```python
from build123d import *

# Parameters (mm, degrees)
SKETCH_1_W                = 300
SKETCH_1_H                = 300
EXTRUDE_1_DEPTH           = 4
EXTRUDE_2_DEPTH           = 76
FILLET_1_R                = 3
CUT_EXTRUDE_1_DEPTH       = 345.818792991
CUT_EXTRUDE_1_DEPTH_BACK  = 345.818792991
SKETCH_3_R                = 3
SKETCH_3_R_2              = 19.5
SKETCH_4_W                = 6
SKETCH_4_H                = 300
EXTRUDE_3_DEPTH           = 76
SKETCH_7_R                = 2
CUT_EXTRUDE_3_DEPTH       = 10
SKETCH_14_W               = 80
SKETCH_14_H               = 30
CUT_EXTRUDE_9_DEPTH       = 20
CUT_EXTRUDE_10_DEPTH      = 345.818792991
CUT_EXTRUDE_10_DEPTH_BACK = 345.818792991
SKETCH_15_R               = 3.5
SKETCH_16_W               = 4
SKETCH_16_H               = 288
EXTRUDE_5_DEPTH           = 9
CHAMFER_3_SIZE            = 50
SKETCH_17_R               = 2.25
SKETCH_17_R_2             = 2.5
CUT_EXTRUDE_11_DEPTH      = 6
SKETCH_18_W               = 137.872576177
SKETCH_18_H               = 47.95567867
SKETCH_18_W_2             = 92.314681441
SKETCH_18_H_2             = 203.212188366
SKETCH_18_W_3             = 138.671837489
SKETCH_18_H_3             = 133.676454294
SKETCH_18_H_4             = 48.754939981
CUT_EXTRUDE_12_DEPTH      = 6
FILLET_4_R                = 3


with BuildPart() as part:
    # Эскиз1 → Бобышка-Вытянуть1 (new body)
    with BuildSketch(Plane(origin=(0, 0, 0), x_dir=(1, 0, 0), z_dir=(0, 1, 0))):
        Rectangle(SKETCH_1_W, SKETCH_1_H)
    extrude(amount=EXTRUDE_1_DEPTH)

    # Эскиз2 → Бобышка-Вытянуть2 (add)
    with BuildSketch(Plane(origin=(0, 4, 0), x_dir=(1, 0, 0), z_dir=(0, 1, 0))):
        Polygon((150, 150), (-144, 150), (-144, 144), (144, 144), (144, -144), (-144, -144), (-144, -150), (150, -150), (150, 0.239524614), align=None)
    extrude(amount=EXTRUDE_2_DEPTH)

    # Скругление1
    fillet_1_edges = [part.edges().sort_by_distance(p)[0] for p in [
        (150, 40, 150),
        (150, 40, -150),
    ]]
    fillet(fillet_1_edges, radius=FILLET_1_R)

    # Эскиз3 → Вырез-Вытянуть1 (cut, two sides: drawn at the far end of the back side and taken through both)
    with BuildSketch(Plane.XY.offset(150).offset(-CUT_EXTRUDE_1_DEPTH_BACK)):
        with Locations((35.45, 56.55)):
            Circle(SKETCH_3_R)
        with Locations((82.55, 56.55)):
            Circle(SKETCH_3_R)
        with Locations((35.45, 9.45)):
            Circle(SKETCH_3_R)
        with Locations((82.55, 9.45)):
            Circle(SKETCH_3_R)
        with Locations((59, 33)):
            Circle(SKETCH_3_R_2)
    extrude(amount=CUT_EXTRUDE_1_DEPTH + CUT_EXTRUDE_1_DEPTH_BACK, mode=Mode.SUBTRACT)

    # Эскиз4 → Бобышка-Вытянуть3 (add)
    with BuildSketch(Plane(origin=(0, 4, 0), x_dir=(1, 0, 0), z_dir=(0, 1, 0))):
        with Locations((-147, 0)):
            Rectangle(SKETCH_4_W, SKETCH_4_H)
    extrude(amount=EXTRUDE_3_DEPTH)

    # Эскиз7 → Вырез-Вытянуть3 (cut)
    with BuildSketch(Plane(origin=(0, 4, 0), x_dir=(1, 0, 0), z_dir=(0, 1, 0))):
        with Locations(Location((127, 82, 0), (0, 0, 270))):
            Circle(SKETCH_7_R)
        with Locations(Location((134, 75, 0), (0, 0, 270))):
            Circle(SKETCH_7_R)
        with Locations(Location((-23, 82, 0), (0, 0, 270))):
            Circle(SKETCH_7_R)
        with Locations(Location((-30, 75, 0), (0, 0, 270))):
            Circle(SKETCH_7_R)
        with Locations(Location((127, -82, 0), (0, 0, 270))):
            Circle(SKETCH_7_R)
        with Locations(Location((134, -75, 0), (0, 0, 270))):
            Circle(SKETCH_7_R)
        with Locations(Location((-30, -75, 0), (0, 0, 270))):
            Circle(SKETCH_7_R)
        with Locations(Location((-23, -82, 0), (0, 0, 270))):
            Circle(SKETCH_7_R)
    extrude(amount=-CUT_EXTRUDE_3_DEPTH, mode=Mode.SUBTRACT)

    # Эскиз14 → Вырез-Вытянуть9 (cut)
    with BuildSketch(Plane(origin=(0, 4, 0), x_dir=(1, 0, 0), z_dir=(0, 1, 0))):
        with Locations((59, 129)):
            Rectangle(SKETCH_14_W, SKETCH_14_H)
        with Locations((59, -129)):
            Rectangle(SKETCH_14_W, SKETCH_14_H)
    extrude(amount=-CUT_EXTRUDE_9_DEPTH, mode=Mode.SUBTRACT)

    # Эскиз15 → Вырез-Вытянуть10 (cut, two sides: drawn at the far end of the back side and taken through both)
    with BuildSketch(Plane.ZY.offset(150).offset(-CUT_EXTRUDE_10_DEPTH_BACK)):
        with Locations((0, 65)):
            Circle(SKETCH_15_R)
        with Locations((125, 65)):
            Circle(SKETCH_15_R)
        with Locations((-125, 65)):
            Circle(SKETCH_15_R)
        with Locations((-125, 15)):
            Circle(SKETCH_15_R)
        with Locations((125, 15)):
            Circle(SKETCH_15_R)
        with Locations((0, 15)):
            Circle(SKETCH_15_R)
    extrude(amount=CUT_EXTRUDE_10_DEPTH + CUT_EXTRUDE_10_DEPTH_BACK, mode=Mode.SUBTRACT)

    # Эскиз16 → Бобышка-Вытянуть5 (add)
    with BuildSketch(Plane(origin=(0, 4, 0), x_dir=(1, 0, 0), z_dir=(0, 1, 0))):
        with Locations((17, 0)):
            Rectangle(SKETCH_16_W, SKETCH_16_H)
    extrude(amount=EXTRUDE_5_DEPTH)

    # Фаска3
    chamfer_3_edges = [part.edges().sort_by_distance(p)[0] for p in [
        (17, 13, -144),
        (17, 13, 144),
    ]]
    chamfer(chamfer_3_edges, length=CHAMFER_3_SIZE)

    # Эскиз17 → Вырез-Вытянуть11 (cut)
    with BuildSketch(Plane(origin=(0, 4, 0), x_dir=(1, 0, 0), z_dir=(0, 1, 0))):
        with Locations(Location((0, 134, 0), (0, 0, 270))):
            Circle(SKETCH_17_R)
        with Locations(Location((0, 104, 0), (0, 0, 270))):
            Circle(SKETCH_17_R)
        with Locations(Location((-64, 134, 0), (0, 0, 270))):
            Circle(SKETCH_17_R)
        with Locations(Location((-64, 104, 0), (0, 0, 270))):
            Circle(SKETCH_17_R)
        with Locations(Location((-128, 134, 0), (0, 0, 270))):
            Circle(SKETCH_17_R)
        with Locations(Location((-128, 104, 0), (0, 0, 270))):
            Circle(SKETCH_17_R)
        with Locations(Location((-128, -104, 0), (0, 0, 90))):
            Circle(SKETCH_17_R)
        with Locations(Location((-128, -134, 0), (0, 0, 90))):
            Circle(SKETCH_17_R)
        with Locations(Location((-64, -104, 0), (0, 0, 90))):
            Circle(SKETCH_17_R)
        with Locations(Location((-64, -134, 0), (0, 0, 90))):
            Circle(SKETCH_17_R)
        with Locations(Location((0, -104, 0), (0, 0, 90))):
            Circle(SKETCH_17_R)
        with Locations(Location((0, -134, 0), (0, 0, 90))):
            Circle(SKETCH_17_R)
        with Locations(Location((-129, 0, 0), (0, 0, 270))):
            Circle(SKETCH_17_R_2)
        with Locations(Location((-59, 0, 0), (0, 0, 270))):
            Circle(SKETCH_17_R_2)
        with Locations(Location((-59, 40, 0), (0, 0, 270))):
            Circle(SKETCH_17_R_2)
        with Locations(Location((-129, 40, 0), (0, 0, 270))):
            Circle(SKETCH_17_R_2)
        with Locations(Location((-59, 80, 0), (0, 0, 270))):
            Circle(SKETCH_17_R_2)
        with Locations(Location((-129, 80, 0), (0, 0, 270))):
            Circle(SKETCH_17_R_2)
        with Locations(Location((-59, -40, 0), (0, 0, 270))):
            Circle(SKETCH_17_R_2)
        with Locations(Location((-129, -40, 0), (0, 0, 270))):
            Circle(SKETCH_17_R_2)
        with Locations(Location((-59, -80, 0), (0, 0, 270))):
            Circle(SKETCH_17_R_2)
        with Locations(Location((-129, -80, 0), (0, 0, 270))):
            Circle(SKETCH_17_R_2)
    extrude(amount=-CUT_EXTRUDE_11_DEPTH, mode=Mode.SUBTRACT)

    # Эскиз18 → Вырез-Вытянуть12 (cut)
    with BuildSketch(Plane(origin=(0, 4, 0), x_dir=(1, 0, 0), z_dir=(0, 1, 0))):
        with Locations((-63.441366575, -113.894736842)):
            Rectangle(SKETCH_18_W, SKETCH_18_H)
        with Locations((73.032502308, -0.699353647)):
            Rectangle(SKETCH_18_W_2, SKETCH_18_H_2)
        with Locations((-68.037119113, -1.698430286)):
            Rectangle(SKETCH_18_W_3, SKETCH_18_H_3)
        with Locations((-63.441366575, 113.495106187)):
            Rectangle(SKETCH_18_W, SKETCH_18_H_4)
    extrude(amount=-CUT_EXTRUDE_12_DEPTH, mode=Mode.SUBTRACT)

    # Скругление4
    fillet_4_edges = [part.edges().sort_by_distance(p)[0] for p in [
        (-144, 42, -144),
        (19, 31.5, -144),
        (144, 42, -144),
        (144, 42, 144),
        (19, 31.5, 144),
        (-144, 42, 144),
        (15, 33.5, -144),
        (15, 33.5, 144),
    ]]
    fillet(fillet_4_edges, radius=FILLET_4_R)


solid = part.part
```
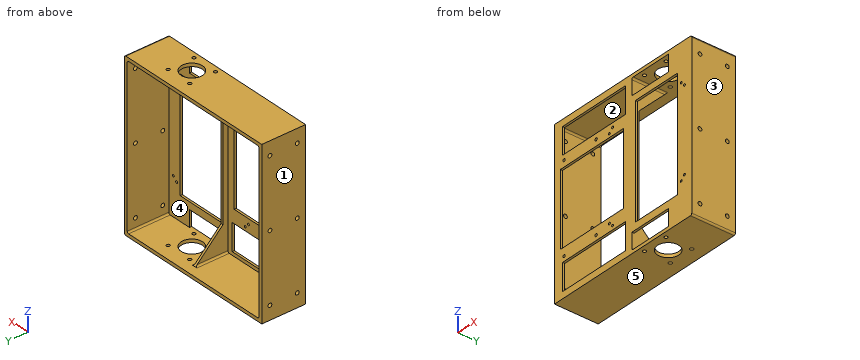
Work out the finished part from the listing and answer in its coordinate system (mm). Face numbers are marked on the shaded views. A direction names the side the tool comes from. Give positions to 0.01 mm unless a question says otherwise; leave off trailing zeros. Write each loop counter-clockwise with the first axis right and the second up, starting at its lowest first coordinate (ties: lowest second). Pieces come first, ordered by that corner, then holes. Notation, with made-up numbers: (5, -40) -> (24, -40) arc R19 cw to (24, -28) -> close; hole circle Ø9 at (23.5, 7). An arc over 180 degrees is marked (long way). Write item = value, one per line.
Q1. A tool of negligible diameter and unlimited length cuts with its end or side. For the marked faces 1 and 2, from which of +Z, -Z, +X, -X, +Y, -Y can it reach the whole face along a straight path? Write none if from no direction.
Computed values:
face_1 = +Z, -Z, -X, +Y, -Y
face_2 = +Y
Q2. Section A-A on x = 107.5 is taken. Determine the outline of the cut face in (y, z).
Computed values:
outline = (0, -150) -> (80, -150) -> (80, -144) -> (4, -144) -> (4, -100.91) -> (0, -100.91) -> close; (0, 102.31) -> (4, 102.31) -> (4, 144) -> (80, 144) -> (80, 150) -> (0, 150) -> close
Q3. Flat-ended cylindrical pins translate along their axes: pin 1 Ø5 at (x, z) = (-30, 75) entering from -Y; pin 2 Ø6.5 at (y, z) = (65, 125) entering from +X; pin 3 Ø1 at (x, z) = (20.5, -28) entering from +Y. Find the tip coordinate at first contact, or state that the pin passes through.
Computed values:
pin_1 = 0
pin_2 = through
pin_3 = 4
Q4. Section C-C on z = -125 is taken. State how many separate pieces and enclosed holes the cut face has, and give its area (3 significant figures).
Computed values:
separate_pieces = 7
enclosed_holes = 0
area = 1,230 mm^2
Q5. Section D-D on x = -10.5 is taken. Determine the outline of the cut face in (y, z), and give its area (3 significant figures).
Computed values:
outline = (0, -150) -> (80, -150) -> (80, -144) -> (4, -144) -> (4, -137.87) -> (0, -137.87) -> close; (0, -89.12) -> (4, -89.12) -> (4, -65.14) -> (0, -65.14) -> close; (0, 68.54) -> (4, 68.54) -> (4, 89.92) -> (0, 89.92) -> close; (0, 137.87) -> (4, 137.87) -> (4, 144) -> (80, 144) -> (80, 150) -> (0, 150) -> close
area = 1,190 mm^2
Q6. For a pull along X with two mould halves and no side action, classify the marked faces 3, 4 and 5 as pulls with the +X half, pulls with the -X half, needs draft (parallel to the pull), parting line crosses it, or undercut.
Computed values:
face_3 = pulls with the +X half
face_4 = undercut
face_5 = needs draft
Q7. Consider line 1 along Y through (x, z) = (-146.5, -125); line 2 along X through (y, z) = (6, 3); line 3 along Y through (x, z) = (82, -146). Determine where each line is inside the solid, lowest interval first.
Computed values:
line_1 = 0 to 11.5, 18.5 to 61.5, 68.5 to 80
line_2 = -150 to -144, 15 to 19, 144 to 150
line_3 = 0 to 6.5, 12.4 to 53.6, 59.5 to 80
